from build123d import *

# Parameters (mm, degrees)
SKETCH2_R           = 25
BOSS_EXTRUDE1_DEPTH = 2
CUT_EXTRUDE1_DEPTH  = 3
CIRPATTERN1_COUNT   = 30
SKETCH5_R           = 8
BOSS_EXTRUDE2_DEPTH = 22


with BuildPart() as part:
    # Sketch2 → Boss-Extrude1 (new body)
    with BuildSketch(Plane(origin=(0, 0, 0), x_dir=(1, 0, 0), z_dir=(0, 1, 0))):
        Circle(SKETCH2_R)
    extrude(amount=BOSS_EXTRUDE1_DEPTH)

    # Sketch1 → Cut-Extrude1 (cut, through all)
    with BuildSketch(Plane(origin=(0, 0, 0), x_dir=(1, 0, 0), z_dir=(0, 1, 0))):
        with BuildLine():
            ThreePointArc((0, 19), (-1.459542881, 21.5), (0, 24))
            ThreePointArc((0, 24), (1.459542881, 21.5), (0, 19))
        make_face()
    cut_extrude1 = extrude(amount=CUT_EXTRUDE1_DEPTH, mode=Mode.SUBTRACT)

    # CirPattern1: Cut-Extrude1 ×30 about axis
    cirpattern1_axis = Axis((0, 0, 0), (0, 1, 0))
    for i in range(1, CIRPATTERN1_COUNT):
        add(cut_extrude1.rotate(cirpattern1_axis, i * 360 / CIRPATTERN1_COUNT), mode=Mode.SUBTRACT)

    # Sketch4 → Revolve1 (revolve)
    with BuildSketch(Plane.XY):
        Polygon((-8, 5), (0, 5), (0, 2), (-9, 2), align=None)
    revolve(axis=Axis((0, 5, 0), (0, -1, 0)))

    # Sketch5 → Boss-Extrude2 (add)
    with BuildSketch(Plane(origin=(0, 5, 0), x_dir=(1, 0, 0), z_dir=(0, 1, 0))):
        Circle(SKETCH5_R)
    extrude(amount=BOSS_EXTRUDE2_DEPTH)


solid = part.part
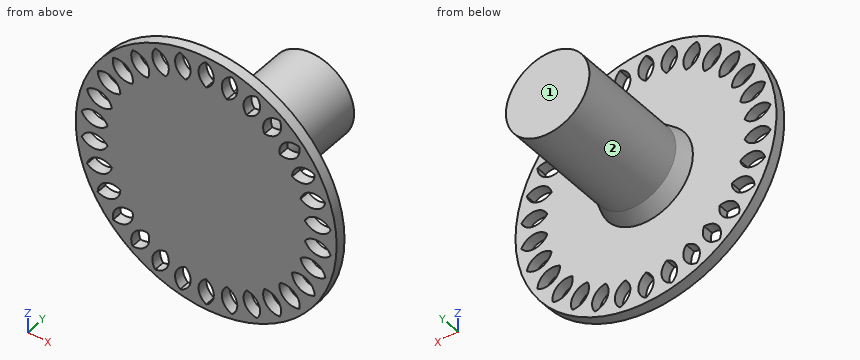
Geometry check sheet. Reference: the model listing, model coordinates, mm. Face numbers are marked on the shaded views. A direction names the side the tool comes from. Round coordinates to 2 decimals unless told otherwise and drop trailing zeros. Write each loop counter-clockwise with the first axis right and the second up, starting at its lowest first coordinate (ties: lowest second). Pieces come first, ordered by that corner, then holes. Notation, with made-up numbers: (68.25, 25.5) - (74.25, 25.5) arc R29 ccw to (74.25, 55.5) - close; hole circle Ø11 at (59.5, 45.25). An arc over 180 degrees is marked (long way). One line per item, written item: value.
1. Cross-section at C-C on y = 23. Record the boundary of the cut face in (x, z), and give its area (3 significant figures).
The answers:
outline: circle Ø16 at (0, 0)
area: 201 mm^2
2. Depth check by flat-ended pin: pin 1 Ø5 at (y, z) = (21.5, 12) entering from -X; pin 2 Ø10 at (x, y) = (-4, 20) entering from -Z; pin 3 Ø1 at (y, z) = (21, -7) entering from +X; pin 4 Ø10 at (x, z) = (-5, 15) entering from +Y. Enter the tip coordinate at first touch or a pass-through.
The answers:
pin 1: passes through
pin 2: stops at z = -8
pin 3: stops at x = 4.66
pin 4: stops at y = 2
3. Set-up check for the marked faces 1 and 2: record each of +Z, -Z, +X, -X, +Y, -Y from which the full face is reachable in a straight line by a thin tool's end or side.
The answers:
face 1: +Z, -Z, +X, -X, +Y
face 2: +Y
4. Cross-section at A-A on x = 12.5. Record the boundary of the cut face in (y, z), and give its area (3 significant figures).
The answers:
outline: (0, -21.65) - (2, -21.65) - (2, -19.13) - (0, -19.13) - close; (0, -15.53) - (2, -15.53) - (2, 15.53) - (0, 15.53) - close; (0, 19.13) - (2, 19.13) - (2, 21.65) - (0, 21.65) - close
area: 72.2 mm^2
5. Scan lines: L1, parallel to X at y = 3, z = 7; L2, parallel to Y at x = -8, z = 9; L3, parallel to Z at x = -1, y = 12.25. Record each from-to range of solid material in increasing order.
The answers:
L1: x = -5.11 to 5.11
L2: y = 0 to 2
L3: z = -7.94 to 7.94
6. Cross-section at B-B on z = 0. Record the boundary of the cut face in (x, y).
The answers:
outline: (-25, 0) - (25, 0) - (25, 2) - (9, 2) - (8, 5) - (8, 27) - (-8, 27) - (-8, 5) - (-9, 2) - (-25, 2) - close
